Autodesk Inventor part; units mm, degrees
ref_plane "YZ Plane" through (0, 0, 0) normal (1, 0, 0) x (0, 1, 0)
ref_plane "XZ Plane" through (0, 0, 0) normal (0, 1, 0) x (-1, 0, 0)
ref_plane "XY Plane" through (0, 0, 0) normal (0, 0, 1) x (1, 0, 0)
sketch "Sketch1" plane through (0, 0, 0) normal (1, 0, 0) x (0, 1, 0)
  line L0 (-17.75, 24) -> (17.75, 24)
  line L1 (17.75, 24) -> (17.75, -24)
  line L2 (17.75, -24) -> (-17.75, -24)
  line L3 (-17.75, -24) -> (-17.75, 24)
  line L4 (-17.75, 24) -> (17.75, -24) construction
  line L5 (17.75, 24) -> (-17.75, -24) construction
  line L6 (17.75, 15) -> (22.75, 15)
  line L7 (22.75, 15) -> (22.75, -15)
  line L8 (22.75, -15) -> (17.75, -15)
  line L9 (17.75, 0) -> (-17.75, 0) construction
  line L10 (0, 24) -> (0, -24)
  arc A0 (17.75, 18) -> (17.75, 15) centre (17.75, 16.5) ccw
  line L11 (17.75, -15) -> (22.75, -15)
  arc A1 (17.75, -15) -> (17.75, -18) centre (17.75, -16.5) ccw
  line L12 (-17.75, 15) -> (-22.75, 15)
  line L13 (-22.75, 15) -> (-22.75, -15)
  line L14 (-22.75, -15) -> (-17.75, -15)
  arc A2 (-17.75, 15) -> (-17.75, 18) centre (-17.75, 16.5) ccw
  arc A3 (-17.75, -18) -> (-17.75, -15) centre (-17.75, -16.5) ccw
  line L15 (17.75, 21) -> (12.75, 21) construction
  line L16 (-10.75, 22.5) -> (10.75, 22.5)
  line L17 (12.358, 17.9707) -> (1.608, 3.4355)
  line L18 (-12.358, 17.9707) -> (-1.608, 3.4355)
  line L19 (1.8124, 1.1893) -> (11.9735, 14.9282)
  line L20 (15.5815, 13.7389) -> (15.5815, -13.7389)
  line L21 (1.8124, -1.1893) -> (11.9735, -14.9282)
  arc A4 (-1.608, 3.4355) -> (1.608, 3.4355) centre (0, 4.6248) ccw
  arc A5 (15.5815, 13.7389) -> (11.9735, 14.9282) centre (13.5815, 13.7389) ccw
  arc A6 (1.8124, 1.1893) -> (1.8124, -1.1893) centre (3.4204, 0) ccw
  arc A7 (11.9735, -14.9282) -> (15.5815, -13.7389) centre (13.5815, -13.7389) ccw
  line L22 (17.75, -21) -> (12.75, -21) construction
  line L23 (12.75, 19.16) -> (12.75, 20.5)
  line L24 (-12.75, 19.16) -> (-12.75, 20.5)
  arc A8 (12.75, 20.5) -> (10.75, 22.5) centre (10.75, 20.5) ccw
  arc A9 (12.358, 17.9707) -> (12.75, 19.16) centre (10.75, 19.16) ccw
  arc A10 (-10.75, 22.5) -> (-12.75, 20.5) centre (-10.75, 20.5) ccw
  arc A11 (-12.75, 19.16) -> (-12.358, 17.9707) centre (-10.75, 19.16) ccw
  circle A12 centre (20.25, 0) radius 1 construction
  line L25 (20.25, 15) -> (20.25, -15) construction
  line L26 (-10.75, -22.5) -> (10.75, -22.5)
  line L27 (12.358, -17.9707) -> (1.608, -3.4355)
  line L28 (-12.358, -17.9707) -> (-1.608, -3.4355)
  arc A13 (1.608, -3.4355) -> (-1.608, -3.4355) centre (0, -4.6248) ccw
  line L29 (12.75, -19.16) -> (12.75, -20.5)
  line L30 (-12.75, -19.16) -> (-12.75, -20.5)
  arc A14 (10.75, -22.5) -> (12.75, -20.5) centre (10.75, -20.5) ccw
  arc A15 (12.75, -19.16) -> (12.358, -17.9707) centre (10.75, -19.16) ccw
  arc A16 (-12.75, -20.5) -> (-10.75, -22.5) centre (-10.75, -20.5) ccw
  arc A17 (-12.358, -17.9707) -> (-12.75, -19.16) centre (-10.75, -19.16) ccw
  point P0 (0, 0)
  point P1 (0, 1.2613)
  point P2 (0.9328, 0)
  point P3 (15.5815, 19.8066)
  point P4 (15.5815, -19.8066)
  point P5 (-12.75, 22.5)
  point P6 (12.75, 22.5)
  point P7 (0, 2.6248)
  point P8 (17.75, -18)
  point P9 (0, 22.5)
  point P10 (12.75, 18.5007)
  point P11 (-12.75, 18.5007)
  point P12 (0, -2.6248)
  point P13 (0, -22.5)
  dimension "d0" = 1.5
  dimension "d1" = 5
  dimension "d2" = 48
  dimension "d3" = 9
  dimension "d4" = 35.5
  dimension "d5" = 5
  dimension "d6" = 1.5
  dimension "d8" = 1.5
  dimension "d9" = 1.5
  dimension "d22" = 2
  dimension "d24" = 2
extrude "Extrusion1" add sketch "Sketch1" along normal blind 5 contours L0 L1 A0 A1 L2 L10 L26 A14 L29 A15 L27 A13 A4 L17 A9 L23 A8 L16 | L6 L7 L8 L1
sketch "Sketch2" plane through (0, 17.75, 24) normal (0, 1, 0) x (1, 0, 0)
  line L0 (0, 45) -> (5, 45)
  line L1 (0, 3) -> (5, 3)
  line L2 (5, 6) -> (5, 0)
  line L3 (5, 48) -> (5, 42)
  line L4 (0, 6) -> (0, 0)
  line L5 (0, 48) -> (0, 42)
  point P0 (0, 3)
  point P1 (0, 3)
  point P2 (0, 3)
  point P3 (0, 45)
  point P4 (2.5, 3)
  point P5 (2.5, 45)
hole "Side-M3" at (2.5, 17.75, -21) at (2.5, 17.75, 21) direction (0, -1, 0) diameter 2.459 end through all
hole "Phi2-H7" at (0, 20.25, 0) direction (1, 0, 0) diameter 2 end through all
chamfer "C0.5" distance 0.5 angle 45 2 edges at (2.5, 22.75, 15) (2.5, 22.75, -15)
mirror "Mirror1" about plane through (0, 0, 2.6248) normal (0, -1, 0)
equation "\"d8\" = d6"
equation "\"d9\" = d6"
equation "\"d17\" = d5"
properties part number "KneeBraceFrame" material "Acetal Resin, Black"
Here's how the part is built. I have some questions about the finished solid (model axes, mm). A direction names the side the tool comes from. Coordinates: 2 decimals unless noted, no trailing zeros. Order: outer loops, then holes, each group sorted by start corner. A loop starts at its lowest first (then second) coordinate and runs counter-clockwise, first axis right, second up. Notation, with made-up numbers: (-19.5, 3) - (-10.5, 3) arc R34 cw to (-10.5, 35) - close; hole circle Ø6 at (-37.75, 62.5). An arc over 180 degrees is marked (long way). Use CSV: the item, a comma, the result in double quotes. Start each with the question number.
1. Suppose I cut it at B-B on y = -13.5. List the corners of the cut face in (x, z) for me, then the cut area to 3 significant figures.
2. Please list where these lines run through material, in increasing order: line 1 (Z direction, x = 4.75, y = 0); line 2 (X direction, y = -13.5, z = 21); line 3 (Y direction, x = 4.05, z = 10). Write a range as from..to.
3. Suppose I cut it at A-A on y = -20.25. List the corners of the cut face in (x, z) for me.
4. I'm going to push flat-ended pins straight in: pin 1 (2 mm diameter, centred on x = 1.5, y = -19.5, fed in from +Z); pin 2 (12 mm diameter, centred on y = 4.5, z = -16, fed in from -X); pin 3 (1.3 mm diameter, centred on x = 2.5, y = 20, fed in from -Z); pin 4 (1.5 mm diameter, centred on x = 2.5, z = -20, fed in from -Y). Where does each tip first touch, or does it pass through?
5. For faces 3 (the face through (2.46, 6.82, -7.96)), 4 (the face through (2, 0, -24)), 5 (the face through (1, -17.75, 22)), 6 (the face through (2, 20, -15)), 7 (the face through (1, 17.75, 20)), which set-ups out of +Z, -Z, +X, -X, +Y, -Y let a thin tool reach every point of the face, with its end or its side?
6. Suppose I cut it at D-D on z = -5.5. List the corners of the cut face in (x, y) for me, then the cut area to 3 significant figures.
7. Suppose I cut it at C-C on x = 2.5. Give the number of separate pieces and of enclosed holes in the cut face, then the cut area to 3 significant figures.
8. If we mould it in two halves opening along X, with no side actions, what happens to faces 1 (the face through (2.971, 15.376, 22.136)), 2 (the face through (2.465, -6.908, 10.601))? For each: +X half, -X half, draft (parallel to the pull), parting line (faces both ways), or undercut.
Output:
1,outline,"(0, -24) - (5, -24) - (5, -15.74) - (0, -15.74) - close; (0, 15.74) - (5, 15.74) - (5, 24) - (0, 24) - close; hole circle Ø2.46 at (2.5, -21); hole circle Ø2.46 at (2.5, 21)"
1,area,"73.1 mm2"
2,line 1,"z = -24..-22.5, -2.62..2.62, 22.5..24"
2,line 2,"x = 0..1.27, 3.73..5"
2,line 3,"y = -22.75..-15.58, -8.33..-6.46, 6.46..8.33, 15.58..22.75"
3,outline,"(0, -15) - (5, -15) - (5, -1) - (0, -1) - close; (0, 1) - (5, 1) - (5, 15) - (0, 15) - close"
4,pin 1,"stops at z = 15"
4,pin 2,"stops at x = 0"
4,pin 3,"stops at z = -15"
4,pin 4,"stops at y = -17.75"
5,face 3,"+X, -X"
5,face 4,"-Z, +X, -X, +Y, -Y"
5,face 5,"+Z, +X, -X, -Y"
5,face 6,"-Z, +X, -X, +Y"
5,face 7,"+Z, +X, -X, +Y"
6,outline,"(0, -22.75) - (5, -22.75) - (5, -15.58) - (0, -15.58) - close; (0, -5) - (5, -5) - (5, -3.13) - (0, -3.13) - close; (0, 3.13) - (5, 3.13) - (5, 5) - (0, 5) - close; (0, 15.58) - (5, 15.58) - (5, 22.75) - (0, 22.75) - close"
6,area,"90.3 mm2"
7,separate pieces,"3"
7,enclosed holes,"4"
7,area,"744 mm2"
8,face 1,"undercut"
8,face 2,"draft"
